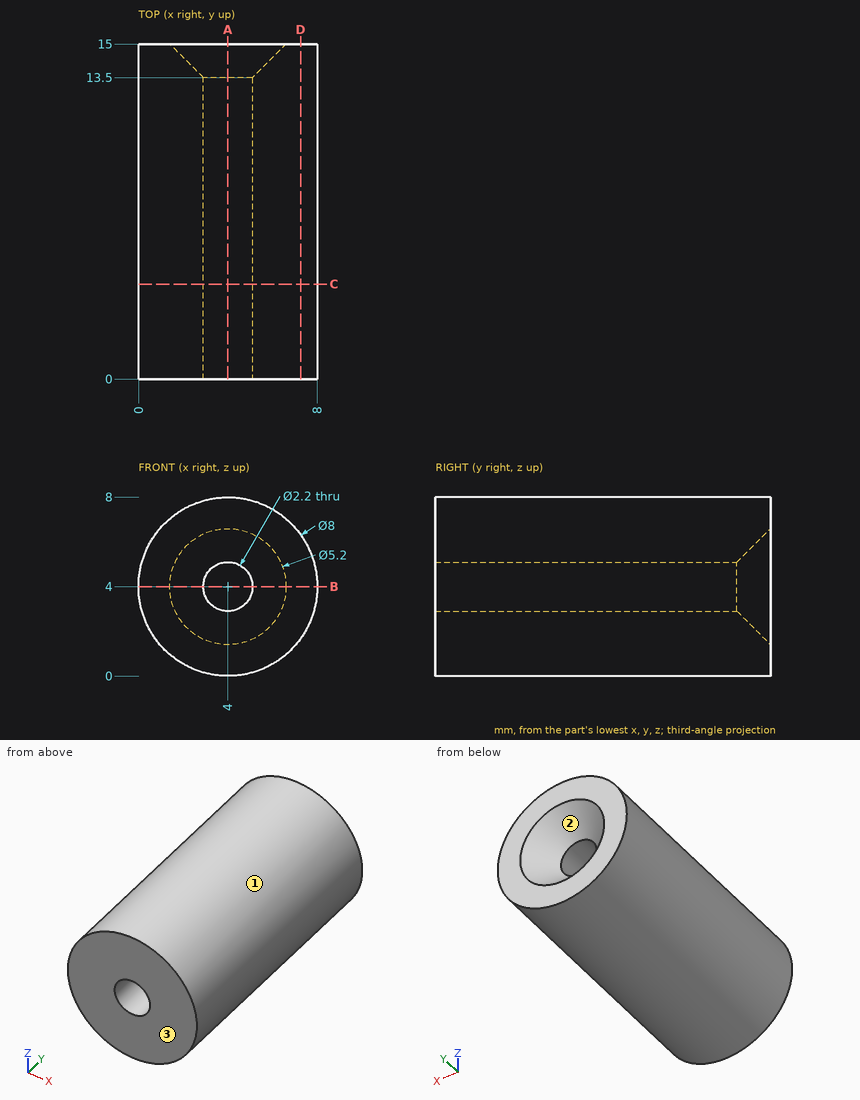
Study the drawing (mm; zero at the part's minimum x, y, z) and answer. Coordinates: 2 decimals unless noted, no trailing zeros. Write each loop counter-clockwise with the first axis right and the second up, starting at its lowest first coordinate (ties: lowest second). Pieces come first, ordered by that corner, then holes. Notation, with made-up numbers: M 85.25,50 L 120.25,50 A23 cw 120.25,66 Z; hole C -20,48 d1. An arc over 180 degrees is marked long. Use one line per item in the form item = value.
Item 1: Find section D-D, the plane x = 7.25. Give the vertices of the cut face in (y, z).
Model answer:
outline = M 0,1.67 L 15,1.67 L 15,6.33 L 0,6.33 Z
Item 2: Given P1, Ø2, axis at y = 2.5, z = 1.5, coming from the -X side; P2, Ø2, axis at x = 4, z = 4, coming from the -Y side; P3, Ø1, axis at y = 6, z = 5.5, coming from the +X side; P4, Ø4, axis at x = 1.5, y = 7.5, coming from the -Z side, each flat-ended and moving along its own axis, determine where each tip first touches the part or whether it passes through.
Model answer:
P1 = 0.29
P2 = through
P3 = 7.87
P4 = 0.03
Item 3: Find section A-A, the plane x = 4. Give the vertices of the cut face in (y, z), plus the area to 4 significant figures.
Model answer:
outline = M 0,0 L 15,0 L 15,1.4 L 13.5,2.9 L 0,2.9 Z; M 0,5.1 L 13.5,5.1 L 15,6.6 L 15,8 L 0,8 Z
area = 84.75 mm2
Item 4: Find section B-B, the plane z = 4. Give the vertices of the cut face in (x, y), plus the area to 4 significant figures.
Model answer:
outline = M 0,0 L 2.9,0 L 2.9,13.5 L 1.4,15 L 0,15 Z; M 5.1,0 L 8,0 L 8,15 L 6.6,15 L 5.1,13.5 Z
area = 84.75 mm2
Item 5: The mould has two halves that part along X. Classify the marked faces 1, 2 and 3: released by +X, released by -X, zero draft, split by the parting line, or undercut.
Model answer:
face_1 = split by the parting line
face_2 = undercut
face_3 = zero draft
Item 6: Find the intervals of material crossed by probe 1 along Z at (x, y) = (4, 4.25); probe 2 along X at (y, z) = (11, 3.75); probe 3 along Z at (x, y) = (3.25, 14.5), in increasing order.
Model answer:
probe_1 = 0 to 2.9, 5.1 to 8
probe_2 = 0.01 to 2.93, 5.07 to 7.99
probe_3 = 0.07 to 2.04, 5.96 to 7.93
Item 7: Find section C-C, the plane y = 4.25. Give the vertices of the cut face in (x, z).
Model answer:
outline = C 4,4 d8; hole C 4,4 d2.2
